```python
from build123d import *

# Parameters (mm, degrees)
F0_W     = 14.6
F0_H     = 15
F0_R     = 3
F1_DEPTH = 7.5
F2_SIZE  = 1
F3_R     = 4
F4_DEPTH = 5.7
F5_W     = 1
F5_H     = 1
F7_SIZE  = 0.5
F8_R     = 2


# Not quite as in the source:
# - a pattern or mirror of a feature is missing from the dataset's text; its kind, count and spacing are read off the source's solid


with BuildPart() as f1:
    # F0 (on Front) → F1 (new body, symmetric)
    with BuildSketch(Plane.XZ):
        Rectangle(F0_W, F0_H)
        Circle(F0_R, mode=Mode.SUBTRACT)
    extrude(amount=F1_DEPTH, both=True)

    # F2
    f2_edges = [f1.edges().sort_by_distance(p)[0] for p in [
        (-3, -7.5, 0),
        (-3, 7.5, 0),
    ]]
    chamfer(f2_edges, length=F2_SIZE)

    # F3 (on face) → F4 (join)
    with BuildSketch(Plane.YZ.offset(7.3)):
        Circle(F3_R)
    f4 = extrude(amount=F4_DEPTH)

    # F4_copies: F4 across plane
    add(f4.mirror(Plane(origin=(0, 0, 0), x_dir=(0, 0, -1), z_dir=(-1, 0, 0))))

    # F5 (on Front) → F6 (revolve, cut)
    with BuildSketch(Plane.XZ):
        with Locations((10.5, 3.5)):
            Rectangle(F5_W, F5_H)
    f6 = revolve(axis=Axis((10.5, 0, 0), (-1, 0, 0)), mode=Mode.SUBTRACT)

    # F6_copies: F6 across plane
    add(f6.mirror(Plane(origin=(0, 0, 0), x_dir=(0, 0, -1), z_dir=(-1, 0, 0))), mode=Mode.SUBTRACT)

    # F7
    f7_edges = [f1.edges().sort_by_distance(p)[0] for p in [
        (13, -4, 0),
        (-13, -4, 0),
    ]]
    chamfer(f7_edges, length=F7_SIZE)

    # F8
    f8_edges = [f1.edges().sort_by_distance(p)[0] for p in [
        (-7.3, 0, 7.5),
        (7.3, 0, 7.5),
        (-7.3, 0, -7.5),
        (7.3, 0, -7.5),
    ]]
    fillet(f8_edges, radius=F8_R)


solid = f1.part
```
Design review of the part built by this model. Coordinates are the model's own, in mm. A direction names the side the tool comes from. Round coordinates to 2 decimals unless told otherwise and drop trailing zeros. Write each loop counter-clockwise with the first axis right and the second up, starting at its lowest first coordinate (ties: lowest second). Pieces come first, ordered by that corner, then holes.
Item 1: We need section A-A on x = 0. Write out the cut boundary in (y, z), and give its area (3 significant figures).
Item 2: The part is to be moulded in two halves that separate along X. For faces 5 (the cylindrical face through (-3, 0, 0)), 6 (the flat face through (0, 0, -7.5)), 7 (the flat face through (-7.3, -2, -4)), say which applies: +X half, -X half, draft (parallel to the pull), parting line (faces both ways), or undercut.
Item 3: Clearance check with a flat-ended pin moving along its axis: pin 1 Ø1.5 at (y, z) = (5.5, -5) entering from +X. State where the tip first meets the part, or that it passes through.
Item 4: We need section B-B on y = 5. Write out the cut boundary in (x, z).
Item 5: For probe 1 along Z at (x, y) = (0, 2); probe 2 along X at (y, z) = (-3, 4.75); probe 3 along Z at (x, y) = (-2.25, 6), list the stretches that pass through material, from the lowest coordinate up.
Item 6: For faces 1 (the cylindrical face through (11.74, 3.815, 1.201)), 2 (the flat face through (10, 3, -1)), 3 (the cylindrical face through (-11.74, 3.815, 1.201)), 4 (the cylindrical face through (-6.7, 0.11, 6.93)), list the 3-axis set-ups (+Z, -Z, +X, -X, +Y, -Y) from which the entire face can be reached by the end or side of a thin tool; tool diameter is ignored.
Item 7: We need section C-C on z = -4.75. Write out the cut boundary in (x, y).
Returned:
1. outline: (-7.5, -7.5) - (7.5, -7.5) - (7.5, -4) - (6.5, -3) - (-6.5, -3) - (-7.5, -4) - close; (-7.5, 4) - (-6.5, 3) - (6.5, 3) - (7.5, 4) - (7.5, 7.5) - (-7.5, 7.5) - close
1. area: 133 mm2
2. face 5: undercut
2. face 6: draft
2. face 7: -X half
3. pin 1: stops at x = 7.3
4. outline: (-7.3, -5.5) arc R2 ccw to (-5.3, -7.5) - (5.3, -7.5) arc R2 ccw to (7.3, -5.5) - (7.3, 5.5) arc R2 ccw to (5.3, 7.5) - (-5.3, 7.5) arc R2 ccw to (-7.3, 5.5) - close; hole circle Ø6 at (0, 0)
5. probe 1: z = -7.5 to -3, 3 to 7.5
5. probe 2: x = -7.3 to 7.3
5. probe 3: z = -7.5 to -1.98, 1.98 to 7.5
6. face 1: +X
6. face 2: none
6. face 3: -X
6. face 4: +Z, -X, +Y, -Y
7. outline: (-7.3, -7.5) - (7.3, -7.5) - (7.3, 7.5) - (-7.3, 7.5) - close
